Autodesk Inventor part; units mm, degrees
ref_plane "YZ Plane" through (0, 0, 0) normal (1, 0, 0) x (0, 1, 0)
ref_plane "XZ Plane" through (0, 0, 0) normal (0, 1, 0) x (-1, 0, 0)
ref_plane "XY Plane" through (0, 0, 0) normal (0, 0, 1) x (1, 0, 0)
sketch "スケッチ1" plane through (0, 0, 0) normal (0, 0, 1) x (1, 0, 0)
  circle A0 centre (0, 0) radius 47.6
  circle A1 centre (0, 0) radius 67.5
  dimension "d0" = 95.2
  dimension "d1" = 135
extrude "押し出し1" add sketch "スケッチ1" along normal blind 10
sketch "スケッチ5" plane through (0, 0, 10) normal (0, 0, 1) x (1, 0, 0)
  circle A0 centre (0, 0) radius 67.5
  circle A1 centre (0, 0) radius 47.6
  circle A2 centre (0, 0) radius 45.5
  dimension "d29" = 91
extrude "押し出し4" add sketch "スケッチ5" along normal blind 1.2 contours A0 | A1
sketch "スケッチ2" plane through (0, 0, 0) normal (0, 0, 1) x (1, 0, 0)
  circle A0 centre (0, 0) radius 62.5
  point P0 (16.1762, 60.3704)
  point P1 (-16.1762, 60.3704)
  point P2 (-44.1942, 44.1942)
  point P3 (-60.3704, 16.1762)
  point P4 (-60.3704, -16.1762)
  point P5 (-44.1942, -44.1942)
  point P6 (-16.1762, -60.3704)
  point P7 (16.1762, -60.3704)
  point P8 (44.1942, -44.1942)
  point P9 (60.3704, -16.1762)
  point P10 (60.3704, 16.1762)
  point P11 (44.1942, 44.1942)
  dimension "d4" = 125
  dimension "d7" = 360
  dimension "d25" = 0
hole "穴1" at (16.1762, 60.3704, 0) at (-16.1762, 60.3704, 0) at (-44.1942, 44.1942, 0) at (-60.3704, 16.1762, 0) at (-60.3704, -16.1762, 0) at (-44.1942, -44.1942, 0) at (-16.1762, -60.3704, 0) at (16.1762, -60.3704, 0) at (44.1942, -44.1942, 0) at (60.3704, -16.1762, 0) at (60.3704, 16.1762, 0) at (44.1942, 44.1942, 0) direction (0, 0, 1) diameter 4.3 end through all
chamfer "面取り2" distance 0.5 angle 45 1 edges at (-47.6, 0, 0)
sketch "スケッチ3" plane through (0, 0, 10) normal (0, 0, 1) x (1, 0, 0)
  circle A0 centre (16.1762, 60.3704) radius 2.15
  circle A1 centre (-16.1762, 60.3704) radius 2.15
  circle A2 centre (0, 0) radius 67.5
  circle A3 centre (0, 0) radius 62.5
  circle A4 centre (-16.1762, 60.3704) radius 5
  circle A5 centre (16.1762, 60.3704) radius 5
  point P0 (11.2987, 61.4702)
  point P1 (17.4703, 65.2)
  point P2 (-17.4703, 65.2)
  point P3 (-20.9502, 58.8841)
properties part number "scara-base3" material "ABS プラスチック"
CAD build for the part. Positions are in the model's coordinates, mm. A direction names the side the tool comes from. Coordinates: 2 decimals unless noted, no trailing zeros. Write each loop counter-clockwise with the first axis right and the second up, starting at its lowest first coordinate (ties: lowest second). Pieces come first, ordered by that corner, then holes. Notation, with made-up numbers: (-28, 84.25) -> (-18, 84.25) arc R18 ccw to (-18, 103.25) -> close; hole circle Ø2 at (71, 28). An arc over 180 degrees is marked (long way). Return JSON: item names as keys, results as strings. Group by question number.
Q1. Which spindle directions (+Z, -Z, +X, -X, +Y, -Y) get a long thin tool onto all of the face, cutting with end or side? Do faces 4 (the face through (-16.27, -62.52, 5.68)), 5 (the face through (-35.083, -32.17, 5.184)). Say none if no direction does.
Q2. Cut at A-A, the plane x = 0. Give the cut face in (y, z).
Q3. Drill centre lines: line 1 (Y direction, x = 0, z = 4.25); line 2 (Y direction, x = 43, z = 8.5); line 3 (X direction, y = -1, z = 8.5). Where is each one in solid material? Low to high.
Q4. Cut at C-C, the plane z = 3.5. State how many separate pieces and enclosed holes the cut face has, then the cut area to 3 significant figures.
Q5. Cut at D-D, the plane x = -52.5. Give the cut face in (y, z), then the cut area to 3 significant figures.
Q6. Pull direction X, two halves, no side cores. Call faces 1 (the face through (45, 20, 0)), 2 (the face through (-53.57, 41.07, 5.52)), 3 (the face through (45, -42.2, 5.7)): released by +X, released by -X, zero draft, split by the parting line, or undercut.
Q7. Flat gauge pins, fed straight in: pin 1 (6 mm diameter, centred on x = -1, z = 5.5, fed in from -Y); pin 2 (4 mm diameter, centred on x = -44.19, y = 44.19, fed in from +Z); pin 3 (6 mm diameter, centred on y = 6.5, z = 7.5, fed in from -X); pin 4 (4 mm diameter, centred on y = 5, z = 6.5, fed in from +X). Where does each tip first touch, or does it go through?
Returned:
{
 "1": {"face 4": "+Z, -Z", "face 5": "-Z"},
 "2": {"outline": "(-67.5, 0) -> (-48.1, 0) -> (-47.6, 0.5) -> (-47.6, 10) -> (-45.5, 10) -> (-45.5, 11.2) -> (-67.5, 11.2) -> close; (45.5, 10) -> (47.6, 10) -> (47.6, 0.5) -> (48.1, 0) -> (67.5, 0) -> (67.5, 11.2) -> (45.5, 11.2) -> close"},
 "3": {"line 1": "y = -67.5 to -47.6, 47.6 to 67.5", "line 2": "y = -52.03 to -45.98, -42.41 to -20.41, 20.41 to 42.41, 45.98 to 52.03", "line 3": "x = -67.49 to -47.59, 47.59 to 67.49"},
 "4": {"separate pieces": "1", "enclosed holes": "13", "area": "7,020 mm2"},
 "5": {"outline": "(-42.43, 0) -> (42.43, 0) -> (42.43, 11.2) -> (-42.43, 11.2) -> close", "area": "950 mm2"},
 "6": {"face 1": "zero draft", "face 2": "split by the parting line", "face 3": "undercut"},
 "7": {"pin 1": "stops at y = -67.5", "pin 2": "passes through", "pin 3": "stops at x = -67.41", "pin 4": "stops at x = 67.43"}
}
